Work out the finished part from the listing and answer in its coordinate system (mm). Coordinates: 2 decimals unless noted, no trailing zeros. Loops run counter-clockwise (first coordinate to the right, second up) from the corner with the lowest first, then second, coordinate; pieces in that order, holes last. Notation, with made-up numbers: M -14,74.25 L 37,74.25 A28 ccw 37,92.25 Z; hole C 62.5,-37 d6. An arc over 180 degrees is marked long. Write each question's results on one line, items separated by ' | '.
```python
from build123d import *

# Parameters (mm, degrees)
F1_DEPTH = 38
F2_W     = 38
F2_H     = 374
F3_DEPTH = 38


with BuildPart() as f1:
    # F0 (on Front) → F1 (new body)
    with BuildSketch(Plane.XZ):
        Polygon((280.465763, 0), (-169.534237, 0), (-131.534237, -38), (242.465763, -38), align=None)
    extrude(amount=F1_DEPTH)


with BuildPart() as f3:
    # F2 (on Front) → F3 (new body)
    with BuildSketch(Plane.XZ):
        with Locations((-266.727887, -67.336804)):
            Rectangle(F2_W, F2_H)
    extrude(amount=F3_DEPTH)


solid = f1.part
```
1) Given pin 1 Ø3 at (y, z) = (-22.5, -4) entering from -X; pin 2 Ø2 at (y, z) = (-25.5, -32.5) entering from -X; pin 3 Ø12 at (y, z) = (-7, -29) entering from +X, each flat-ended and moving along its own axis, determine where each tip first touches the part or whether it passes through.
Check result:
pin 1: x = -167.03 | pin 2: x = -138.03 | pin 3: x = 257.47
2) Find section A-A, the plane y = -26.5. Give the vertices of the cut face in (x, z).
Check result:
outline: M -169.53,0 L -131.53,-38 L 242.47,-38 L 280.47,0 Z
3) Straight lines are drawn through the part: probe 1 along X at (y, z) = (-19, -33); probe 2 along Z at (x, y) = (250.5, -11); probe 3 along X at (y, z) = (-10, -5). For each, find the intervals that lie inside material, in ascending order. Write a range as [from, to].
Check result:
probe 1: [-136.53, 247.47] | probe 2: [-29.97, 0] | probe 3: [-164.53, 275.47]
4) Find section B-B, the plane z = -23. Give the vertices of the cut face in (x, y), and give its area (3 significant figures).
Check result:
outline: M -146.53,-38 L 257.47,-38 L 257.47,0 L -146.53,0 Z | area: 15,400 mm^2
